from build123d import *

# Parameters (mm, degrees)
BOSS_EXTRUDE1_DEPTH = 1.6
FILLET1_R           = 0.5
FILLET2_R           = 0.25
FILLET3_R           = 0.15
CUT_EXTRUDE1_DEPTH  = 0.3
FILLET4_R           = 4
SKETCH3_R           = 1
CUT_EXTRUDE2_DEPTH  = 42.249281937
FILLET5_R           = 4
FILLET6_R           = 1
FILLET7_R           = 0.15


with BuildPart() as part:
    # Sketch1 → Boss-Extrude1 (new body)
    with BuildSketch(Plane.XY):
        with BuildLine():
            Line((0, 0), (0, 6.2))
            Line((0, 6.2), (25.416876048, 6.2))
            ThreePointArc((25.416876048, 6.2), (34.077130086, 4.922813233), (42, 1.2))
            Line((42, 1.2), (12, 1.2))
            Line((12, 1.2), (10.8, 0))
            Line((10.8, 0), (0, 0))
        make_face()
    extrude(amount=BOSS_EXTRUDE1_DEPTH)

    # Fillet1
    fillet1_edges = [part.edges().sort_by_distance(p)[0] for p in [
        (42, 1.2, 0.8),
    ]]
    fillet(fillet1_edges, radius=FILLET1_R)

    # Fillet2
    fillet2_edges = [part.edges().sort_by_distance(p)[0] for p in [
        (12, 1.2, 0.8),
        (10.8, 0, 0.8),
    ]]
    fillet(fillet2_edges, radius=FILLET2_R)

    # Fillet3
    fillet3_edges = [part.edges().sort_by_distance(p)[0] for p in [
        (12.708438024, 6.2, 1.6),
        (33.228210707, 5.16520414, 0),
        (33.228210707, 5.16520414, 1.6),
        (0, 3.1, 1.6),
        (40.732026425, 1.569811089, 0),
        (40.732026425, 1.569811089, 1.6),
        (11.4, 0.6, 0),
        (11.4, 0.6, 1.6),
        (26.176413207, 1.2, 0),
        (10.792117467, 0.019030117, 0),
        (26.176413207, 1.2, 1.6),
        (10.792117467, 0.019030117, 1.6),
        (12.007882533, 1.180969883, 0),
        (12.007882533, 1.180969883, 1.6),
        (5.348223305, 0, 1.6),
        (0, 3.1, 0),
        (12.708438024, 6.2, 0),
        (5.348223305, 0, 0),
    ]]
    fillet(fillet3_edges, radius=FILLET3_R)

    # Sketch2 → Cut-Extrude1 (cut)
    with BuildSketch(Plane(origin=(0, 0, 0), x_dir=(-1, 0, 0), z_dir=(0, 0, -1))):
        with BuildLine():
            Line((-16.416876048, 5.55), (-28.416876048, 5.55))
            ThreePointArc((-28.416876048, 5.55), (-22.416876048, 4.297727085), (-16.416876048, 5.55))
        make_face()
    extrude(amount=-CUT_EXTRUDE1_DEPTH, mode=Mode.SUBTRACT)

    # Fillet4
    # the kernel refuses this fillet: 4 mm, written as the material it adds along each edge
    with BuildSketch(Plane(origin=(22.416876048, 19.297727085, 0.3), x_dir=(0.6169459509621767, -0.7870055232279983, 0), z_dir=(0.7870055232279983, 0.6169459509621767, 0))) as fillet4_piece_1_section:
        with BuildLine():
            CenterArc((13.480131585, 4), FILLET4_R, 270, 22.331645009)
            Line((13.480131585, 0), (13.480131585, -0.08))
            Line((13.480131585, -0.08), (15, -0.08))
            Line((15, -0.08), (15.08, 0))
            ThreePointArc((15.08, 0), (15.08, 0.15), (15.030397368, 0.226))
            Line((15.030397368, 0.226), (15, 0.3))
        make_face()
    fillet4_piece_1 = revolve(axis=Axis((22.416876048, 19.297727085, 0.3), (0, 0, -1)), revolution_arc=76.186906047, mode=Mode.PRIVATE)
    fillet4_piece_1 = split(fillet4_piece_1, bisect_by=Plane(origin=(22.416876137, 5.55, 0.246369344), z_dir=(0, -1, 0)), keep=Keep.TOP, mode=Mode.PRIVATE)
    add(fillet4_piece_1)

    # Sketch3 → Cut-Extrude2 (cut, through all)
    with BuildSketch(Plane(origin=(0, 0, 0), x_dir=(-1, 0, 0), z_dir=(0, 0, -1))):
        with Locations((-3.45, 3.4)):
            Circle(SKETCH3_R)
    extrude(amount=-CUT_EXTRUDE2_DEPTH, mode=Mode.SUBTRACT)

    # Fillet5
    # the kernel refuses this fillet: 4 mm, written as the material it takes off along each edge
    with BuildSketch(Plane(origin=(4, 4, 0), x_dir=(0, -1, 0), z_dir=(1, 0, 0))) as fillet5_piece_1:
        with BuildLine():
            CenterArc((3.85, -0.15), 0.15, 0, 90)
            Line((4, -0.15), (4, 0))
            Line((4, 0), (3.85, 0))
        make_face()
    revolve(axis=Axis((4, 4, 0), (0, 0, -1)), revolution_arc=90, mode=Mode.SUBTRACT)
    with BuildSketch(Plane(origin=(4, 4, 1.6), x_dir=(-1, 0, 0), z_dir=(0, 1, 0))) as fillet5_piece_2:
        with BuildLine():
            CenterArc((3.85, -0.15), 0.15, 0, 90)
            Line((4, -0.15), (4, 0))
            Line((4, 0), (3.85, 0))
        make_face()
    revolve(axis=Axis((4, 4, 1.6), (0, 0, 1)), revolution_arc=90, mode=Mode.SUBTRACT)
    with BuildSketch(Plane(origin=(0, 0, 0), x_dir=(0, 1, 0), z_dir=(0, 0, 1))) as fillet5_piece_3:
        with BuildLine():
            CenterArc((FILLET5_R, -FILLET5_R), FILLET5_R, 90, 90)
            Line((0, -FILLET5_R), (0, 0))
            Line((0, 0), (FILLET5_R, 0))
        make_face()
    extrude(amount=1.6, mode=Mode.SUBTRACT)

    # Fillet6
    # the kernel refuses this fillet: 1 mm, written as the material it takes off along each edge
    with BuildSketch(Plane(origin=(1, 5.2, 0), x_dir=(-1, 0, 0), z_dir=(0, -1, 0))) as fillet6_piece_1:
        with BuildLine():
            CenterArc((0.85, -0.15), 0.15, 0, 90)
            Line((1, -0.15), (1, 0))
            Line((1, 0), (0.85, 0))
        make_face()
    revolve(axis=Axis((1, 5.2, 0), (0, 0, -1)), revolution_arc=90, mode=Mode.SUBTRACT)
    with BuildSketch(Plane(origin=(1, 5.2, 1.6), x_dir=(0, 1, 0), z_dir=(1, 0, 0))) as fillet6_piece_2:
        with BuildLine():
            CenterArc((0.85, -0.15), 0.15, 0, 90)
            Line((1, -0.15), (1, 0))
            Line((1, 0), (0.85, 0))
        make_face()
    revolve(axis=Axis((1, 5.2, 1.6), (0, 0, 1)), revolution_arc=90, mode=Mode.SUBTRACT)
    with BuildSketch(Plane(origin=(0, 6.2, 0), x_dir=(0, -1, 0), z_dir=(0, 0, 1))) as fillet6_piece_3:
        with BuildLine():
            CenterArc((FILLET6_R, FILLET6_R), FILLET6_R, 180, 90)
            Line((0, FILLET6_R), (0, 0))
            Line((0, 0), (FILLET6_R, 0))
        make_face()
    extrude(amount=1.6, mode=Mode.SUBTRACT)

    # Fillet7
    fillet7_edges = [part.edges().sort_by_distance(p)[0] for p in [
        (4.45, 3.4, 1.6),
        (4.45, 3.4, 0),
    ]]
    fillet(fillet7_edges, radius=FILLET7_R)


solid = part.part
Geometry check sheet. Reference: the model listing, model coordinates, mm. A direction names the side the tool comes from. Round coordinates to 2 decimals unless told otherwise and drop trailing zeros. Loops run counter-clockwise (first coordinate to the right, second up) from the corner with the lowest first, then second, coordinate; pieces in that order, holes last. Notation, with made-up numbers: (61, 77.25) -> (88, 77.25) arc R7 ccw to (88, 87.25) -> close; hole circle Ø9 at (85.5, 23). An arc over 180 degrees is marked (long way). Answer as a JSON object with one key per item and string values. Group by question number.
Item 1: Set-up check for faces 4 (the face through (13, 6.2, 1)), 5 (the face through (26, 1.2, 1)): record each of +Z, -Z, +X, -X, +Y, -Y from which the full face is reachable in a straight line by a thin tool's end or side.
Item 2: Cross-section at A-A, the plane z = 1.1. Record the cut outline in (x, y), plus the area to 3 significant figures.
Item 3: Release check for a two-part mould opening along X. For faces 1 (the face through (0, 5, 1)), 2 (the face through (16, 3, 0)), 3 (the face through (3.667, 2.424, 0.791)) record: pulls with the +X half, pulls with the -X half, needs draft (parallel to the pull), parting line crosses it, or undercut.
Item 4: Thickness scan on line 1 along Y through (x, z) = (17.5, 0.9); line 2 along Y through (x, z) = (3.45, 0.5); line 3 along X through (y, z) = (3, 0.8). Record the ranges inside material, lowest first.
Determined:
{
 "1": {"face 4": "+Z, -Z, +X, -X, +Y", "face 5": "+Z, -Z, +X, -Y"},
 "2": {"outline": "(0, 4) arc R4 ccw to (4, 0) -> (10.7, 0) arc R0.25 ccw to (10.87, 0.07) -> (11.93, 1.13) arc R0.25 cw to (12.1, 1.2) -> (40.25, 1.2) arc R0.5 ccw to (40.5, 2.13) arc R30 ccw to (25.42, 6.2) -> (1, 6.2) arc R1 ccw to (0, 5.2) -> close; hole circle Ø2 at (3.45, 3.4)", "area": "190 mm²"},
 "3": {"face 1": "pulls with the -X half", "face 2": "needs draft", "face 3": "undercut"},
 "4": {"line 1": "y = 1.2 to 6.2", "line 2": "y = 0.04 to 2.4, 4.4 to 6.2", "line 3": "x = 0.13 to 2.53, 4.37 to 38.9"}
}
